from build123d import *

# Parameters (mm, degrees)
SKETCH1_W                           = 105
SKETCH1_H                           = 35
BOSS_EXTRUDE1_DEPTH                 = 14
CUT_EXTRUDE1_DEPTH                  = 0.5
CUT_EXTRUDE2_START                  = -0.5
CUT_EXTRUDE2_DEPTH                  = 0.5
FILLET1_R                           = 4
FILLET2_R                           = 1
ESQUISSE1_R                         = 2
ENL_V_MAT_EXTRU_1_DEPTH             = 0.25
ENL_V_MAT_EXTRU_1_DIRECTION_2_REACH = 109.012
ENL_V_MAT_EXTRU_4_DEPTH             = 0.25


with BuildPart() as part:
    # Sketch1 → Boss-Extrude1 (new body)
    with BuildSketch(Plane(origin=(0, 0, -15), x_dir=(-1, 0, 0), z_dir=(0, 0, -1))):
        Rectangle(SKETCH1_W, SKETCH1_H)
    extrude(amount=-BOSS_EXTRUDE1_DEPTH)

    # Sketch2 → Cut-Extrude1 (cut)
    with BuildSketch(Plane(origin=(52.5, 0, 0), x_dir=(0, 0, -1), z_dir=(1, 0, 0))):
        with BuildLine():
            Line((2.75, 9.125), (2.75, -9.125))
            ThreePointArc((2.75, -9.125), (3.921572875, -11.953427125), (6.75, -13.125))
            Line((6.75, -13.125), (9.25, -13.125))
            ThreePointArc((9.25, -13.125), (12.078427125, -11.953427125), (13.25, -9.125))
            Line((13.25, -9.125), (13.25, 9.125))
            ThreePointArc((13.25, 9.125), (12.078427125, 11.953427125), (9.25, 13.125))
            Line((9.25, 13.125), (6.75, 13.125))
            ThreePointArc((6.75, 13.125), (3.921572875, 11.953427125), (2.75, 9.125))
        make_face()
    extrude(amount=-CUT_EXTRUDE1_DEPTH, mode=Mode.SUBTRACT)

    # Sketch3 → Cut-Extrude2 (cut)
    with BuildSketch(Plane.ZY.offset(52.5).offset(CUT_EXTRUDE2_START)):
        with BuildLine():
            Line((-6.75, 13.125), (-9.25, 13.125))
            ThreePointArc((-9.25, 13.125), (-12.078427125, 11.953427125), (-13.25, 9.125))
            Line((-13.25, 9.125), (-13.25, -9.125))
            ThreePointArc((-13.25, -9.125), (-12.078427125, -11.953427125), (-9.25, -13.125))
            Line((-9.25, -13.125), (-6.75, -13.125))
            ThreePointArc((-6.75, -13.125), (-3.921572875, -11.953427125), (-2.75, -9.125))
            Line((-2.75, -9.125), (-2.75, 9.125))
            ThreePointArc((-2.75, 9.125), (-3.921572875, 11.953427125), (-6.75, 13.125))
        make_face()
    extrude(amount=CUT_EXTRUDE2_DEPTH, mode=Mode.SUBTRACT)

    # Fillet1
    # the kernel refuses this fillet: 4 mm, written as the material it takes off along each edge
    with BuildSketch(Plane(origin=(-52.5, -27.5, -15), x_dir=(0, 0, 1), z_dir=(0, 1, 0)), Plane(origin=(52.5, 27.5, -15), x_dir=(0, 0, 1), z_dir=(0, -1, 0))) as fillet1_piece_1:
        with BuildLine():
            CenterArc((FILLET1_R, FILLET1_R), FILLET1_R, 180, 90)
            Line((0, FILLET1_R), (0, 0))
            Line((0, 0), (FILLET1_R, 0))
        make_face()
    extrude(amount=55, mode=Mode.SUBTRACT)
    with BuildSketch(Plane(origin=(-52.5, -27.5, -1), x_dir=(0, 0, -1), z_dir=(0, 1, 0)), Plane(origin=(52.5, 27.5, -1), x_dir=(0, 0, -1), z_dir=(0, -1, 0))) as fillet1_piece_2:
        with BuildLine():
            CenterArc((FILLET1_R, -FILLET1_R), FILLET1_R, 90, 90)
            Line((0, -FILLET1_R), (0, 0))
            Line((0, 0), (FILLET1_R, 0))
        make_face()
    extrude(amount=55, mode=Mode.SUBTRACT)

    # Fillet2
    fillet2_edges = [part.edges().sort_by_distance(p)[0] for p in [
        (0, -17.5, -15),
        (0, 17.5, -15),
        (-52.5, 17.5, -8),
        (0, 17.5, -1),
        (52.5, 17.5, -8),
        (51.328427125, 17.5, -2.171572875),
        (51.328427125, 17.5, -13.828427125),
        (-51.328427125, 17.5, -2.171572875),
        (-51.328427125, 17.5, -13.828427125),
        (-52.5, -17.5, -8),
        (52.5, -17.5, -8),
        (0, -17.5, -1),
        (51.328427125, -17.5, -2.171572875),
        (51.328427125, -17.5, -13.828427125),
        (-51.328427125, -17.5, -2.171572875),
        (-51.328427125, -17.5, -13.828427125),
    ]]
    fillet(fillet2_edges, radius=FILLET2_R)

    # Esquisse1 → Enlèv. mat.-Extru.1 (cut)
    with BuildSketch(Plane(origin=(52, 0, 0), x_dir=(0, 0, -1), z_dir=(1, 0, 0))):
        with Locations(Location((5.75, 12.5, 0), (0, 0, 198.094122224))):
            Circle(ESQUISSE1_R)
        with Locations(Location((10.25, 12.5, 0), (0, 0, 161.790043136))):
            Circle(ESQUISSE1_R)
    extrude(amount=-ENL_V_MAT_EXTRU_1_DEPTH, mode=Mode.SUBTRACT)

    # Esquisse1 → Enlèv. mat.-Extru.1 direction 2 (cut, up to next)
    with BuildSketch(Plane(origin=(52, 0, 0), x_dir=(0, 0, -1), z_dir=(1, 0, 0)), mode=Mode.PRIVATE) as enl_v_mat_extru_1_direction_2_sk1:
        with Locations(Location((5.75, 12.5, 0), (0, 0, 198.094122224))):
            Circle(ESQUISSE1_R)
    enl_v_mat_extru_1_direction_2_tool1 = extrude(enl_v_mat_extru_1_direction_2_sk1.sketch, amount=ENL_V_MAT_EXTRU_1_DIRECTION_2_REACH, mode=Mode.PRIVATE) & part.part
    # Esquisse1 → Enlèv. mat.-Extru.1 direction 2 (cut, up to next)
    with BuildSketch(Plane(origin=(52, 0, 0), x_dir=(0, 0, -1), z_dir=(1, 0, 0)), mode=Mode.PRIVATE) as enl_v_mat_extru_1_direction_2_sk2:
        with Locations(Location((10.25, 12.5, 0), (0, 0, 161.790043136))):
            Circle(ESQUISSE1_R)
    enl_v_mat_extru_1_direction_2_tool2 = extrude(enl_v_mat_extru_1_direction_2_sk2.sketch, amount=ENL_V_MAT_EXTRU_1_DIRECTION_2_REACH, mode=Mode.PRIVATE) & part.part
    add(enl_v_mat_extru_1_direction_2_tool1.solids().sort_by_distance((52, 12.5, -5.75))[0], mode=Mode.SUBTRACT)
    add(enl_v_mat_extru_1_direction_2_tool2.solids().sort_by_distance((52, 12.5, -10.25))[0], mode=Mode.SUBTRACT)

    # Esquisse2 → Enlèv. mat.-Extru.4 (cut)
    with BuildSketch(Plane(origin=(52.5, 0, 0), x_dir=(0, 0, -1), z_dir=(1, 0, 0))):
        with BuildLine():
            ThreePointArc((7.425, 14.928608635), (8, 14.5), (8.575, 14.928608635))
            ThreePointArc((8.575, 14.928608635), (9.75, 15.1), (8.575, 15.271391365))
            ThreePointArc((8.575, 15.271391365), (8, 15.7), (7.425, 15.271391365))
            ThreePointArc((7.425, 15.271391365), (6.25, 15.1), (7.425, 14.928608635))
        make_face()
    extrude(amount=-ENL_V_MAT_EXTRU_4_DEPTH, mode=Mode.SUBTRACT)


solid = part.part
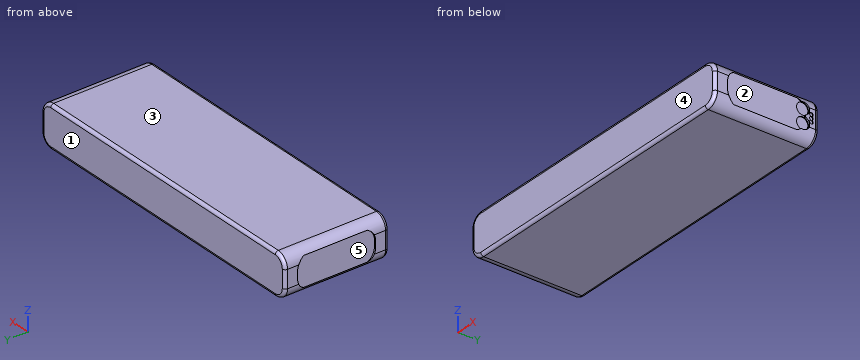
The listing builds one solid part. Answer for the finished solid, in the listing's coordinates (mm). Face numbers are marked on the shaded views. A direction names the side the tool comes from. Coordinates: 2 decimals unless noted, no trailing zeros. Order: outer loops, then holes, each group sorted by start corner. A loop starts at its lowest first (then second) coordinate and runs counter-clockwise, first axis right, second up. Notation, with made-up numbers: (67, 18) -> (95, 18) arc R24 cw to (95, 37) -> close; hole circle Ø5 at (-9, 14). An arc over 180 degrees is marked (long way). Answer in a Markdown table with one row per item. Add a question column.
Item 1: Find section A-A (y = 2). Write down the section's boundary in (x, z), then the cut area to 3 significant figures.
Item 2: Each of these flat-tipped pins is pushed along its axis until it touches: P1, Ø5, axis at y = -2, z = -8, coming from the +X side; P2, Ø1.2, axis at y = 12, z = -9.5, coming from the +X side; P3, Ø5, axis at y = 5.5, z = -8.5, coming from the -X side. Where does it stop, or does it pass through?
Item 3: Determine the mould class of the marked faces 1, 2 and 3 for opening direction Y: +Y half, -Y half, draft (parallel to the pull), parting line (faces both ways), or undercut.
Item 4: Find the intervals of material crossed by L1, parallel to Z at x = 51.9, y = 12.5; L2, parallel to Z at x = 51.95, y = 12.5; L3, parallel to Y at x = 52.3, z = -6.85 (3 decimals), in increasing order. Write a range as from..to.
Item 5: Which of the six approach directions +Z, -Z, +X, -X, +Y, -Y give full straight-line access (tool end or side, diameter ignored) to the marked faces 4 and 5?
Result set:
| question | item | result |
|---|---|---|
| 1 | outline | (-52, -12.94) arc R4 ccw to (-48.5, -15) -> (48.5, -15) arc R4 ccw to (52, -12.94) -> (52, -3.06) arc R4 ccw to (48.5, -1) -> (-48.5, -1) arc R4 ccw to (-52, -3.06) -> close |
| 1 | area | 1,450 mm² |
| 2 | P1 | stops at x = 52 |
| 2 | P2 | stops at x = 51.75 |
| 2 | P3 | stops at x = -52 |
| 3 | face 1 | +Y half |
| 3 | face 2 | undercut |
| 3 | face 3 | draft |
| 4 | L1 | z = -13.11..-12.25, -8.25..-7.75, -3.75..-2.89 |
| 4 | L2 | z = -13.02..-12.25, -8.25..-7.75, -3.75..-2.98 |
| 4 | L3 | y = -17.1..-13.125, 14.17..14.5, 15.7..17.1 |
| 5 | face 4 | +Z, -Z, +X, -X, -Y |
| 5 | face 5 | -X |
